```python
from build123d import *

# Parameters (mm, degrees)
SKETCH1_W               = 222.123
SKETCH1_H               = 254.783638074
SKETCH1_R               = 14.2875
BOSS_EXTRUDE1_DEPTH     = 1.5875
SKETCH4_R               = 2.8067
CUT_EXTRUDE1_DEPTH      = 170.014355888
SKETCH5_R               = 1.5875
CUT_EXTRUDE2_DEPTH      = 170.014355888
SKETCH6_W               = 222.123
SKETCH6_H               = 1.5875
BOSS_EXTRUDE2_DEPTH     = 50.8
SKETCH7_W               = 101.6
SKETCH7_H               = 50.8
CUT_EXTRUDE3_DEPTH      = 210.975001632
SKETCH8_R               = 14.2875
CUT_EXTRUDE5_DEPTH      = 210.975001632
SKETCH9_R               = 2.15
CUT_EXTRUDE6_DEPTH      = 210.975001632
SKETCH10_W              = 57.15
SKETCH10_H              = 50.8
CUT_EXTRUDE7_DEPTH      = 210.975001632
CUT_EXTRUDE8_DEPTH      = 210.975001632
FILLET2_R               = 25.4
CUT_EXTRUDE9_DEPTH      = 210.975001632
CUT_EXTRUDE10_DEPTH     = 210.975001632
CUT_EXTRUDE11_DEPTH     = 210.975001632
CUT_EXTRUDE12_DEPTH     = 210.975001632
SKETCH16_R              = 1.27
CUT_EXTRUDE13_DEPTH     = 210.975001632
F_1_4_CLEARANCE_HOLE1_D = 7.14248


with BuildPart() as part:
    # Sketch1 → Boss-Extrude1 (new body)
    with BuildSketch(Plane(origin=(0, 0, 0), x_dir=(1, 0, 0), z_dir=(0, 1, 0))):
        Rectangle(SKETCH1_W, SKETCH1_H)
        with Locations(Location((9.4615, -78.750819037, 0), (0, 0, 270))):
            Circle(SKETCH1_R, mode=Mode.SUBTRACT)
        with Locations(Location((45.4025, -16.499180963, 0), (0, 0, 270))):
            Circle(SKETCH1_R, mode=Mode.SUBTRACT)
        with Locations(Location((-62.4205, -78.750819037, 0), (0, 0, 270))):
            Circle(SKETCH1_R, mode=Mode.SUBTRACT)
    extrude(amount=BOSS_EXTRUDE1_DEPTH)

    # Sketch4 → Cut-Extrude1 (cut, through all)
    with BuildSketch(Plane(origin=(0, 0, 0), x_dir=(-1, 0, 0), z_dir=(0, -1, 0))):
        with Locations(Location((59.692539866, 117.866819037, 0), (0, 0, 90))):
            Circle(SKETCH4_R)
        with Locations(Location((59.692539866, 22.616819037, 0), (0, 0, 90))):
            Circle(SKETCH4_R)
        with Locations(Location((-6.733539866, 117.866819037, 0), (0, 0, 90))):
            Circle(SKETCH4_R)
        with Locations(Location((-6.733539866, 22.616819037, 0), (0, 0, 90))):
            Circle(SKETCH4_R)
    extrude(amount=-CUT_EXTRUDE1_DEPTH, mode=Mode.SUBTRACT)

    # Sketch5 → Cut-Extrude2 (cut, through all)
    with BuildSketch(Plane.XZ):
        with Locations(Location((59.770116522, -91.195174152, 0), (0, 0, 270))):
            Circle(SKETCH5_R)
    extrude(amount=-CUT_EXTRUDE2_DEPTH, mode=Mode.SUBTRACT)

    # Sketch6 → Boss-Extrude2 (add)
    with BuildSketch(Plane.XY.offset(127.391819037)):
        with Locations((0, 0.79375)):
            Rectangle(SKETCH6_W, SKETCH6_H)
    extrude(amount=BOSS_EXTRUDE2_DEPTH)

    # Sketch7 → Cut-Extrude3 (cut, through all)
    with BuildSketch(Plane(origin=(0, 0, 0), x_dir=(-1, 0, 0), z_dir=(0, -1, 0))):
        with Locations((-60.2615, -152.791819037)):
            Rectangle(SKETCH7_W, SKETCH7_H)
    extrude(amount=-CUT_EXTRUDE3_DEPTH, mode=Mode.SUBTRACT)

    # Sketch8 → Cut-Extrude5 (cut, through all)
    with BuildSketch(Plane(origin=(0, 1.5875, 0), x_dir=(1, 0, 0), z_dir=(0, 1, 0))):
        with Locations(Location((-19.1135, -149.616819037, 0), (0, 0, 270))):
            Circle(SKETCH8_R)
    extrude(amount=-CUT_EXTRUDE5_DEPTH, mode=Mode.SUBTRACT)

    # Sketch9 → Cut-Extrude6 (cut, through all)
    with BuildSketch(Plane(origin=(0, 1.5875, 0), x_dir=(1, 0, 0), z_dir=(0, 1, 0))):
        with Locations(Location((-17.801836865, -125.840471629, 0), (0, 0, 270))):
            Circle(SKETCH9_R)
        with Locations(Location((2.133252432, -138.86457893, 0), (0, 0, 270))):
            Circle(SKETCH9_R)
        with Locations(Location((0.821589297, -162.640926338, 0), (0, 0, 270))):
            Circle(SKETCH9_R)
        with Locations(Location((-20.425163135, -173.393166445, 0), (0, 0, 270))):
            Circle(SKETCH9_R)
        with Locations(Location((-40.360252432, -160.369059145, 0), (0, 0, 270))):
            Circle(SKETCH9_R)
        with Locations(Location((-39.048589297, -136.592711737, 0), (0, 0, 270))):
            Circle(SKETCH9_R)
    extrude(amount=-CUT_EXTRUDE6_DEPTH, mode=Mode.SUBTRACT)

    # Sketch10 → Cut-Extrude7 (cut, through all)
    with BuildSketch(Plane(origin=(0, 1.5875, 0), x_dir=(1, 0, 0), z_dir=(0, 1, 0))):
        with Locations((-82.4865, 64.242728021)):
            Rectangle(SKETCH10_W, SKETCH10_H)
    extrude(amount=-CUT_EXTRUDE7_DEPTH, mode=Mode.SUBTRACT)

    # Sketch11 → Cut-Extrude8 (cut, through all)
    with BuildSketch(Plane(origin=(0, 1.5875, 0), x_dir=(1, 0, 0), z_dir=(0, 1, 0))):
        with BuildLine():
            Line((-9.5885, -178.191819037), (9.4615, -178.191819037))
            Line((9.4615, -178.191819037), (9.4615, -159.141819037))
            ThreePointArc((9.4615, -159.141819037), (3.881884182, -172.612203219), (-9.5885, -178.191819037))
        make_face()
    extrude(amount=-CUT_EXTRUDE8_DEPTH, mode=Mode.SUBTRACT)

    # Fillet2
    fillet2_edges = [part.edges().sort_by_distance(p)[0] for p in [
        (9.4615, 0.79375, 127.391819037),
    ]]
    fillet(fillet2_edges, radius=FILLET2_R)

    # Sketch12 → Cut-Extrude9 (cut, through all)
    with BuildSketch(Plane(origin=(0, 1.5875, 0), x_dir=(1, 0, 0), z_dir=(0, 1, 0))):
        with BuildLine():
            Line((111.0615, -51.191819037), (111.0615, -127.391819037))
            Line((111.0615, -127.391819037), (34.8615, -127.391819037))
            ThreePointArc((34.8615, -127.391819037), (88.743036726, -105.073355764), (111.0615, -51.191819037))
        make_face()
    extrude(amount=-CUT_EXTRUDE9_DEPTH, mode=Mode.SUBTRACT)

    # Sketch13 → Cut-Extrude10 (cut, through all)
    with BuildSketch(Plane(origin=(0, 1.5875, 0), x_dir=(1, 0, 0), z_dir=(0, 1, 0))):
        with BuildLine():
            Line((60.2615, 127.391819037), (111.0615, 127.391819037))
            Line((111.0615, 127.391819037), (111.0615, 76.591819037))
            ThreePointArc((111.0615, 76.591819037), (96.182524484, 112.512843522), (60.2615, 127.391819037))
        make_face()
    extrude(amount=-CUT_EXTRUDE10_DEPTH, mode=Mode.SUBTRACT)

    # Sketch14 → Cut-Extrude11 (cut, through all)
    with BuildSketch(Plane(origin=(0, 1.5875, 0), x_dir=(1, 0, 0), z_dir=(0, 1, 0))):
        with BuildLine():
            Line((-85.6615, 127.391819037), (-111.0615, 127.391819037))
            Line((-111.0615, 127.391819037), (-111.0615, 101.991819037))
            ThreePointArc((-111.0615, 101.991819037), (-103.622012242, 119.95233128), (-85.6615, 127.391819037))
        make_face()
    extrude(amount=-CUT_EXTRUDE11_DEPTH, mode=Mode.SUBTRACT)

    # Sketch15 → Cut-Extrude12 (cut, through all)
    with BuildSketch(Plane(origin=(0, 1.5875, 0), x_dir=(1, 0, 0), z_dir=(0, 1, 0))):
        with BuildLine():
            Line((-111.0615, -127.391819037), (-111.0615, -178.191819037))
            Line((-111.0615, -178.191819037), (-60.2615, -178.191819037))
            ThreePointArc((-60.2615, -178.191819037), (-96.182524484, -163.312843522), (-111.0615, -127.391819037))
        make_face()
    extrude(amount=-CUT_EXTRUDE12_DEPTH, mode=Mode.SUBTRACT)

    # Sketch16 → Cut-Extrude13 (cut, through all)
    with BuildSketch(Plane.XZ):
        with Locations(Location((-85.6615, -108.341819037, 0), (0, 0, 270))):
            Circle(SKETCH16_R)
        with Locations(Location((-79.3115, 13.091819037, 0), (0, 0, 270))):
            Circle(SKETCH16_R)
        with Locations(Location((-72.9615, 140.091819037, 0), (0, 0, 270))):
            Circle(SKETCH16_R)
        with Locations(Location((72.9615, 75.808180963, 0), (0, 0, 270))):
            Circle(SKETCH16_R)
        with Locations(Location((85.6615, -25.791819037, 0), (0, 0, 270))):
            Circle(SKETCH16_R)
        with Locations(Location((15.8115, -51.191819037, 0), (0, 0, 270))):
            Circle(SKETCH16_R)
    extrude(amount=-CUT_EXTRUDE13_DEPTH, mode=Mode.SUBTRACT)

    # 1/4 Clearance Hole1 (through all)
    with Locations(Plane(origin=(0, 1.5875, 0), x_dir=(1, 0, 0), z_dir=(0, 1, 0))):
        with Locations((-85.6615, 108.341819037), (-79.3115, -13.091819037), (-72.9615, -140.091819037), (72.9615, -75.808180963), (85.6615, 25.791819037), (59.770116522, 91.195174152), (15.8115, 51.191819037)):
            Hole(F_1_4_CLEARANCE_HOLE1_D / 2)


solid = part.part
```
The model under review builds one solid part; all positions refer to its coordinate system, in mm. Round coordinates to 2 decimals unless told otherwise and drop trailing zeros. Order: outer loops, then holes, each group sorted by start corner. A loop starts at its lowest first (then second) coordinate and runs counter-clockwise, first axis right, second up.
Item 1: Add section A-A, the plane y = 0.65. Count the separate pieces of the cut face and the enclosed holes in it, and give its area (3 significant figures).
Working result:
separate pieces: 1
enclosed holes: 21
area: 54,300 mm2
Item 2: Draft analysis for pull direction Z (two halves, no side actions). For faces 1 (the flat face through (-2, 0, 23)), 2 (the cylindrical face through (16.586, 0.783, -47.706)), 3 (the cylindrical face through (-103.82, 0.8, -119.75)), state which applies: released by +Z, released by -Z, zero draft, split by the parting line, or undercut.
Working result:
face 1: zero draft
face 2: undercut
face 3: released by -Z
Item 3: Add section B-B, the plane z = -82.5. State the section outline as (x, y) points, and give its area (3 significant figures).
Working result:
outline: (-53.91, 0) - (110.72, 0) - (110.72, 1.59) - (-53.91, 1.59) - close
area: 261 mm2
Item 4: To check wall thickness, follow probe 1 along Z at (x, y) = (-70, 0.9); probe 2 along Z at (x, y) = (-86.5, 1.15); probe 3 along Z at (x, y) = (-63.5, 1.4). State the ranges of each line that lie inside material, in increasing order.
Working result:
probe 1: z = -127.39 to -89.64, -38.84 to 66.64, 90.86 to 138.1, 142.09 to 177.25
probe 2: z = -127.38 to -111.81, -104.87 to -89.64, -38.84 to 170.89
probe 3: z = -127.39 to -89.64, -38.84 to 64.5, 93 to 178.09
Item 5: For pin 1 (0.8 mm diameter, centred on y = 0.5, z = 155.5, fed in from +X), flat-tipped, find the tip position at first contact; note if it passes through.
Working result:
pin 1: stops at x = 9.46
Item 6: Add section C-C, the plane x = 96.5. State the section outline as (y, z) points, and give its area (3 significant figures).
Working result:
outline: (0, -112.19) - (1.59, -112.19) - (1.59, 95.99) - (0, 95.99) - close
area: 330 mm2
